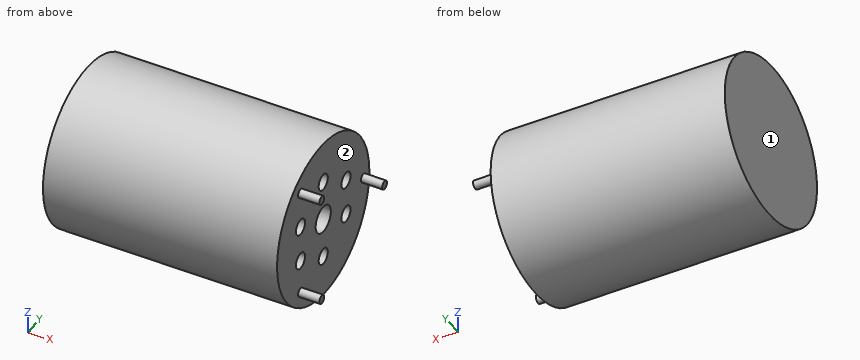
Autodesk Inventor part; units mm, degrees
ref_plane "YZ Plane" through (0, 0, 0) normal (1, 0, 0) x (0, 1, 0)
ref_plane "XZ Plane" through (0, 0, 0) normal (0, 1, 0) x (-1, 0, 0)
ref_plane "XY Plane" through (0, 0, 0) normal (0, 0, 1) x (1, 0, 0)
sketch "Sketch1" plane through (0, 0, 0) normal (1, 0, 0) x (0, 1, 0)
  circle A0 centre (0, 0) radius 9.6564
extrude "Extrusion1" add sketch "Sketch1" along normal blind 15.24
sketch "Sketch2" plane through (15.24, 0, 0) normal (1, 0, 0) x (0, 0, -1)
  circle A0 centre (0, 0) radius 6.5454
  circle A1 centre (0, 0) radius 1.5875
  circle A2 centre (-4.7625, 0) radius 0.9525
  circle A3 centre (2.3204, 4.7625) radius 0.9525
  circle A4 centre (4.7625, 0) radius 0.9525
  circle A5 centre (2.3204, -4.7625) radius 0.9525
  circle A6 centre (-2.0084, -4.7625) radius 0.9525
  circle A7 centre (-2.0084, 4.7625) radius 0.9525
  circle A8 centre (0, 8.2286) radius 0.508
  circle A9 centre (-5.715, -5.715) radius 0.508
  circle A10 centre (5.715, -5.715) radius 0.508
  dimension "d3" = 1.905
  dimension "d5" = 1.905
  dimension "d6" = 1.905
  dimension "d7" = 1.905
  dimension "d8" = 1.905
  dimension "d9" = 1.905
  dimension "d10" = 1.016
  dimension "d11" = 1.016
  dimension "d12" = 1.016
extrude "Extrusion2" cut sketch "Sketch2" against normal blind 10.16 contours A1 | A2 | A3 | A4 | A5 | A6 | A7
sketch "Sketch3" plane through (15.24, 0, 0) normal (1, 0, 0) x (0, 0, -1)
  circle A0 centre (0, 8.3846) radius 0.508
  circle A1 centre (-6.35, -4.7625) radius 0.508
  circle A2 centre (6.35, -4.7625) radius 0.508
  point P0 (0, 0)
  dimension "d15" = 1.016
  dimension "d16" = 1.016
  dimension "d17" = 1.016
extrude "Extrusion3" add sketch "Sketch3" along normal blind 2.54
sketch "Sketch4" plane through (0, 0, 0) normal (-1, 0, 0) x (0, 0, 1)
  circle A0 centre (0, 0) radius 9.6564
extrude "Extrusion4" add sketch "Sketch4" along normal blind 12.7
properties part number "DC SUBMERSIBLE PUMP"
Check sheet for the modelled part. Datum: model origin and axes. Units: mm. Face numbers are marked on the shaded views. Round coordinates to 2 decimals unless told otherwise and drop trailing zeros. Loops run counter-clockwise (first coordinate to the right, second up) from the corner with the lowest first, then second, coordinate; pieces in that order, holes last. Notation, with made-up numbers: (-7, -37.5) - (20, -37.5) arc R33 cw to (20, -6.5) - close; hole circle Ø1 at (-23, -39.75). An arc over 180 degrees is marked (long way). Answer as CSV lines item,"result". Start each with the question number.
Item 1: Release check for a two-part mould opening along X. For the marked faces 1 and 2 record: +X half, -X half, draft (parallel to the pull), parting line (faces both ways), or undercut.
Item 2: Scan lines: line 1 (Z direction, x = 14.5, y = 5.5); line 2 (X direction, y = 3.75, z = 7.75); line 3 (Z direction, x = 13, y = 0.5). Record each from-to range of solid material in increasing order. Write a range as [from, to].
Item 3: Section check A-A (z = -6.35). Record the boundary of the cut face in (x, y), and give its area (3 significant figures).
Item 4: Section check B-B (x = -2.5). Record the boundary of the cut face in (y, z).
Item 5: Depth check by flat-ended pin: P1, Ø1.5, axis at y = -5, z = -2, coming from the +X side; P2, Ø0.6, axis at y = 4.5, z = 2, coming from the +X side; P3, Ø2, axis at x = -4, z = -3.5, coming from the +Y side. Enter the tip coordinate at first touch or a pass-through.
Item 6: Section check C-C (x = 14). Record the boundary of the cut face in (y, z) (1 decimal).
Report:
1,face 1,"-X half"
1,face 2,"+X half"
2,line 1,"z = [-7.94, -2.92], [-1.72, 1.41], [2.61, 7.94]"
2,line 2,"x = [-12.7, 15.24]"
2,line 3,"z = [-9.64, -5.57], [-3.95, -1.51], [1.51, 3.95], [5.57, 9.64]"
3,outline,"(-12.7, -7.27) - (15.24, -7.27) - (15.24, -5.27) - (17.78, -5.27) - (17.78, -4.25) - (15.24, -4.25) - (15.24, 7.27) - (-12.7, 7.27) - close"
3,area,"409 mm2"
4,outline,"circle Ø19.31 at (0, 0)"
5,P1,"stops at x = 15.24"
5,P2,"stops at x = 5.08"
5,P3,"stops at y = 9.33"
6,outline,"circle Ø19.3 at (0, 0); hole circle Ø1.9 at (-4.8, -2.3); hole circle Ø1.9 at (-4.8, 2); hole circle Ø3.2 at (0, 0); hole circle Ø1.9 at (0, -4.8); hole circle Ø1.9 at (0, 4.8); hole circle Ø1.9 at (4.8, -2.3); hole circle Ø1.9 at (4.8, 2)"
